For this review, use the dimensioned drawing (mm, ordinates from the lowest corner) and the shaded views. A direction names the side the tool comes from. Coordinates: 2 decimals unless noted, no trailing zeros. Write each loop counter-clockwise with the first axis right and the second up, starting at its lowest first coordinate (ties: lowest second). Pieces come first, ordered by that corner, then holes.
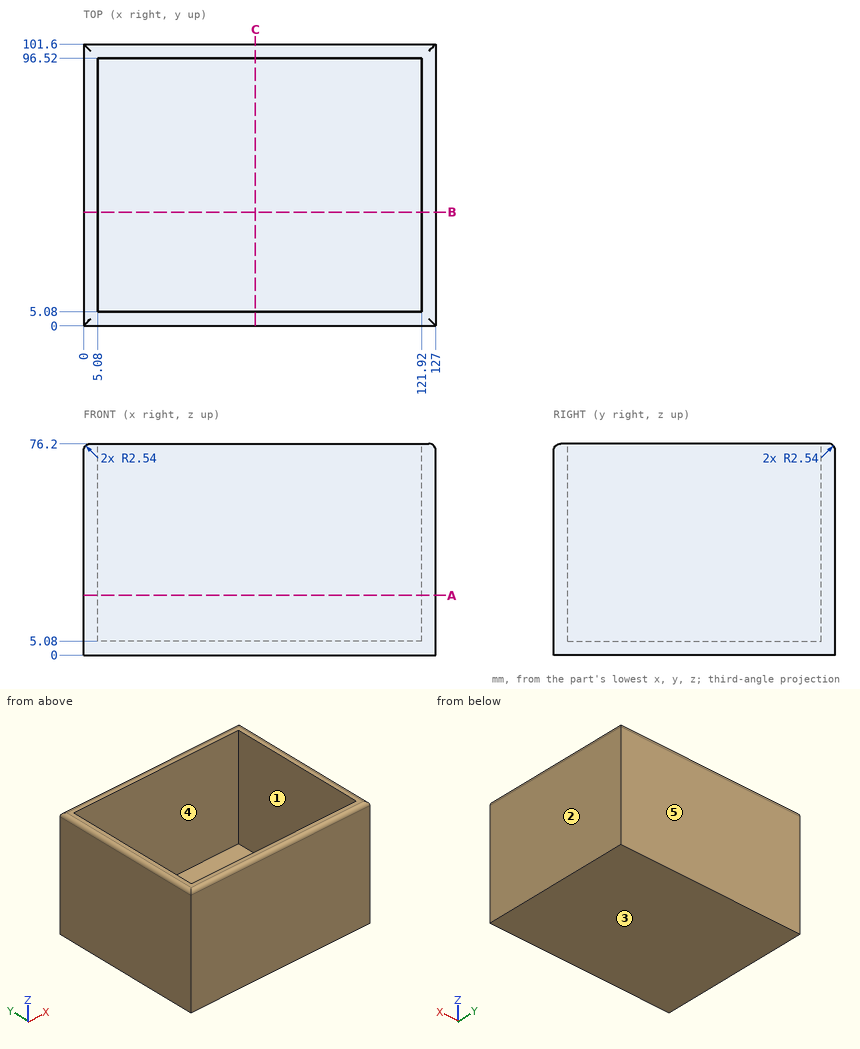
Item 1: Mouldability with a two-part tool opening along X and no side actions: class the marked faces 1, 2 and 3 as pulls with the +X half, pulls with the -X half, needs draft (parallel to the pull), parting line crosses it, or undercut.
Solved:
face 1: undercut
face 2: pulls with the +X half
face 3: needs draft
Item 2: Machinability: for the marked faces 4 and 5, which of the approach directions +Z, -Z, +X, -X, +Y, -Y give a long, thin tool a straight path to every point of the face, cutting with its end or side? Answer none if there is none.
Solved:
face 4: +Z
face 5: +Z, -Z, +X, -X, +Y
Item 3: To check wall thickness, follow line 1 along X through (y, z) = (42, 59); line 2 along Y through (x, z) = (57, 26); line 3 along Z through (x, y) = (44.5, 45.5). State the ranges of each line that lie inside material, in increasing order.
Solved:
line 1: x = 0 to 5.08, 121.92 to 127
line 2: y = 0 to 5.08, 96.52 to 101.6
line 3: z = 0 to 5.08
Item 4: Take a section at A-A, the plane z = 21.5. Write out the cut boundary in (x, y).
Solved:
outline: (0, 0) - (127, 0) - (127, 101.6) - (0, 101.6) - close; hole (5.08, 5.08) - (121.92, 5.08) - (121.92, 96.52) - (5.08, 96.52) - close
Item 5: For pin 1 (4 mm diameter, centred on x = 37.5, y = 53.5, fed in from -Z), flat-tipped, find the tip position at first contact; note if it passes through.
Solved:
pin 1: stops at z = 0
Item 6: Take a section at B-B, the plane y = 41. Write out the cut boundary in (x, z), plus the area to 3 significant figures.
Solved:
outline: (0, 0) - (127, 0) - (127, 73.66) arc R2.54 ccw to (124.46, 76.2) - (121.92, 76.2) - (121.92, 5.08) - (5.08, 5.08) - (5.08, 76.2) - (2.54, 76.2) arc R2.54 ccw to (0, 73.66) - close
area: 1,360 mm2
Item 7: Take a section at C-C, the plane x = 62. Write out the cut boundary in (y, z), plus the area to 3 significant figures.
Solved:
outline: (0, 0) - (101.6, 0) - (101.6, 73.66) arc R2.54 ccw to (99.06, 76.2) - (96.52, 76.2) - (96.52, 5.08) - (5.08, 5.08) - (5.08, 76.2) - (2.54, 76.2) arc R2.54 ccw to (0, 73.66) - close
area: 1,240 mm2
